Could you check a few things on this model? Use its own coordinates, in mm. A direction names the side the tool comes from. Coordinates: 2 decimals unless noted, no trailing zeros. Loops run counter-clockwise (first coordinate to the right, second up) from the corner with the lowest first, then second, coordinate; pieces in that order, holes last. Notation, with made-up numbers: (-30, 20.5) -> (-4, 20.5) arc R26 ccw to (-4, 49.5) -> close; hole circle Ø8 at (38, 23). An arc over 180 degrees is marked (long way). One line per question, with ' | ' between items.
from build123d import *

# Parameters (mm, degrees)
SKETCH1_R           = 8.15
BOSS_EXTRUDE1_DEPTH = 5
SKETCH3_W           = 6
SKETCH3_H           = 4
BOSS_EXTRUDE2_DEPTH = 10
SKETCH4_R           = 1.6
CUT_EXTRUDE1_DEPTH  = 10


with BuildPart() as part:
    # Sketch1 → Boss-Extrude1 (new body)
    with BuildSketch(Plane.XY):
        with BuildLine():
            Line((30, 0), (-30, 0))
            Line((-30, 0), (-30, 5))
            Line((-30, 5), (-22.076055104, 16.485922475))
            ThreePointArc((-22.076055104, 16.485922475), (-9.989658142, 21.089074765), (-1.684442299, 11.174772352))
            Line((-1.684442299, 11.174772352), (1.684442299, 11.174772352))
            ThreePointArc((1.684442299, 11.174772352), (9.989658142, 21.089074765), (22.076055104, 16.485922475))
            Line((22.076055104, 16.485922475), (30, 5))
            Line((30, 5), (30, 0))
        make_face()
        with Locations((-12.8, 10.299057219)):
            Circle(SKETCH1_R, mode=Mode.SUBTRACT)
        with Locations(Location((12.8, 10.299057219, 0), (0, 0, 180))):
            Circle(SKETCH1_R, mode=Mode.SUBTRACT)
    extrude(amount=BOSS_EXTRUDE1_DEPTH)

    # Sketch3 → Boss-Extrude2 (add)
    with BuildSketch(Plane.XY.offset(5)):
        with Locations((-27, 2)):
            Rectangle(SKETCH3_W, SKETCH3_H)
        with Locations((27, 2)):
            Rectangle(SKETCH3_W, SKETCH3_H)
    extrude(amount=BOSS_EXTRUDE2_DEPTH)

    # Sketch4 → Cut-Extrude1 (cut)
    with BuildSketch(Plane(origin=(0, 4, 0), x_dir=(1, 0, 0), z_dir=(0, 1, 0))):
        with Locations(Location((-27, -12, 0), (0, 0, 270))):
            Circle(SKETCH4_R)
        with Locations(Location((27, -12, 0), (0, 0, 270))):
            Circle(SKETCH4_R)
    extrude(amount=-CUT_EXTRUDE1_DEPTH, mode=Mode.SUBTRACT)


solid = part.part
1) If we section it at A-A on z = 6: Please give me the cut outline in (x, y), and give its area (3 significant figures).
Data:
outline: (-30, 0) -> (-24, 0) -> (-24, 4) -> (-30, 4) -> close; (24, 0) -> (30, 0) -> (30, 4) -> (24, 4) -> close | area: 48.0 mm²
2) On a 3-axis mill with a long thin cutter (end or side, diameter ignored), from which of +Z, -Z, +X, -X, +Y, -Y can I reach the whole of each face in a straight line? I mean faces 1 (the face through (24, 2, 10)), 2 (the face through (0, 11.175, 2)), 3 (the face through (27, 2, 15)), 4 (the face through (27, 4, 10)), 5 (the face through (-14.567, 2.343, 2.465)). Say none if no direction works.
Data:
face 1: +Z, +Y, -Y | face 2: +Z, -Z, +Y | face 3: +Z, +X, -X, +Y, -Y | face 4: +Z, +X, -X, +Y | face 5: +Z, -Z
3) We'd pull the mould along X, two halves only. Please class faces 6 (the face through (28.08, 2.03, 10.82)), 7 (the face through (0, 0, 4)), 8 (the face through (-30, 2, 7)), 9 (the face through (-25.92, 2.03, 10.82)): pulls with the +X half, pulls with the -X half, needs draft (parallel to the pull), parting line crosses it, or undercut.
Data:
face 6: undercut | face 7: needs draft | face 8: pulls with the -X half | face 9: undercut
4) If we section it at C-C on z = 12: Please give me the cut outline in (x, y), and give its area (3 significant figures).
Data:
outline: (-30, 0) -> (-28.6, 0) -> (-28.6, 4) -> (-30, 4) -> close; (-25.4, 0) -> (-24, 0) -> (-24, 4) -> (-25.4, 4) -> close; (24, 0) -> (25.4, 0) -> (25.4, 4) -> (24, 4) -> close; (28.6, 0) -> (30, 0) -> (30, 4) -> (28.6, 4) -> close | area: 22.4 mm²
5) If we section it at B-B on x = 12.8: Please give me the cut outline in (y, z), and give its area (3 significant figures).
Data:
outline: (0, 0) -> (2.15, 0) -> (2.15, 5) -> (0, 5) -> close; (18.45, 0) -> (21.45, 0) -> (21.45, 5) -> (18.45, 5) -> close | area: 25.7 mm²
6) If we section it at D-D on y = 9.25: Please give me the cut outline in (x, z).
Data:
outline: (-27.07, 0) -> (-20.88, 0) -> (-20.88, 5) -> (-27.07, 5) -> close; (-4.72, 0) -> (4.72, 0) -> (4.72, 5) -> (-4.72, 5) -> close; (20.88, 0) -> (27.07, 0) -> (27.07, 5) -> (20.88, 5) -> close
7) I need wall thicknesses on line 1 along X through (y, z) = (3.25, 12); line 2 along Y through (x, z) = (-12.8, 1.85); line 3 along X through (y, z) = (15.5, 3.5). Which ranges of each line are inside material? Lowest first, please. Write a range as from..to.
Data:
line 1: -30..-28.6, -25.4..-24, 24..25.4, 28.6..30 | line 2: 0..2.15, 18.45..21.45 | line 3: -22.76..-19.07, -6.53..-2.94, 2.94..6.53, 19.07..22.76
8) I'm going to push flat-ended pins straight in: pin 1 Ø6 at (x, z) = (0.5, 5) entering from +Y; pin 2 Ø6.5 at (x, z) = (-26, 11) entering from +Y; pin 3 Ø3 at (y, z) = (10.5, 1.5) entering from +X; pin 4 Ø5 at (x, z) = (27, 12) entering from -Y. Where does each tip first touch, or does it pass through?
Data:
pin 1: y = 16.45 | pin 2: y = 4 | pin 3: x = 27.24 | pin 4: y = 0
